Verification items for the finished model (mm, model axes). Face numbers are marked on the shaded views. A direction names the side the tool comes from. Round coordinates to 2 decimals unless told otherwise and drop trailing zeros. Order: outer loops, then holes, each group sorted by start corner. A loop starts at its lowest first (then second) coordinate and runs counter-clockwise, first axis right, second up. Notation, with made-up numbers: (-30.75, -6.75) -> (3.25, -6.75) arc R24 cw to (3.25, 28.25) -> close; hole circle Ø11 at (-26, -2). An arc over 180 degrees is marked (long way). Return JSON: item names as keys, results as strings. Group by question number.
1) Section check C-C on x = 25. Enter the section's corners in (y, z), plus the area to 3 significant figures.
2) Section check D-D on z = 32.5. Enter the section's corners in (x, y), plus the area to 3 significant figures.
3) Scan lines: L1, parallel to X at y = 47, z = 0; L2, parallel to Y at x = -43, z = -38; L3, parallel to X at y = 21, z = 3. Record each from-to range of solid material in increasing order.
4) Section check B-B on y = 12. Enter the section's corners in (x, z).
5) Section check A-A on z = 0. Enter the section's corners in (x, y), plus the area to 3 significant figures.
6) Draft check along Z on the marked faces 1, 2 and 3. Enter one of: pulls with the +Z half, pulls with the -Z half, needs draft (parallel to the pull), parting line crosses it, or undercut.
7) Depth check by flat-ended pin: pin 1 (12 mm diameter, centred on y = 33.5, z = 42.5, fed in from +X); pin 2 (19 mm diameter, centred on x = 68, y = 12.5, fed in from -Z); pin 3 (8 mm diameter, centred on x = 74, z = -18.5, fed in from +Y). Enter the tip coordinate at first touch or a pass-through.
8) Tool access check on the marked faces 4, 5, 6, 7 and 8. Record the directions out of +Z, -Z, +X, -X, +Y, -Y that give a thin tool (end or side, any length) a straight path to the whole face; none if there is none.
```python
from build123d import *

# Parameters (mm, degrees)
SKETCH1_R          = 11
BASE_DEPTH         = 24
SKETCH2_R          = 36
SKETCH2_R_2        = 14
TOP_CYLINDER_DEPTH = 38
SIDE_ARMS_DEPTH    = 56


with BuildPart() as part:
    # Sketch1 → base (new body)
    with BuildSketch(Plane(origin=(0, 0, 0), x_dir=(1, 0, 0), z_dir=(0, 1, 0))):
        with BuildLine():
            Line((-28, -50.793700397), (28, -50.793700397))
            ThreePointArc((28, -50.793700397), (41.012193309, -41.012193309), (50.793700397, -28))
            Line((50.793700397, -28), (88, -28))
            ThreePointArc((88, -28), (116, 0), (88, 28))
            Line((88, 28), (50.793700397, 28))
            ThreePointArc((50.793700397, 28), (41.012193309, 41.012193309), (28, 50.793700397))
            Line((28, 50.793700397), (-28, 50.793700397))
            ThreePointArc((-28, 50.793700397), (-58, 0), (-28, -50.793700397))
        make_face()
        with Locations(Location((88, 0, 0), (0, 0, 270))):
            Circle(SKETCH1_R, mode=Mode.SUBTRACT)
    extrude(amount=BASE_DEPTH)

    # Sketch2 → top cylinder (add)
    with BuildSketch(Plane(origin=(0, 24, 0), x_dir=(1, 0, 0), z_dir=(0, 1, 0))):
        with Locations(Location((0, 0, 0), (0, 0, 270))):
            Circle(SKETCH2_R)
        with Locations(Location((0, 0, 0), (0, 0, 270))):
            Circle(SKETCH2_R_2, mode=Mode.SUBTRACT)
    extrude(amount=TOP_CYLINDER_DEPTH)

    # 3DSketch1 → side arms (add)
    with BuildSketch(Plane(origin=(28, 24, 50.793700397), x_dir=(0, 0, -1), z_dir=(1, 0, 0))):
        Polygon((0, 0), (28.166283399, 23.634318012), (28.166283399, 0), align=None)
        Polygon((101.587400794, 0), (73.421117395, 23.634318012), (73.421117395, 0), align=None)
    extrude(amount=-SIDE_ARMS_DEPTH)


solid = part.part
```
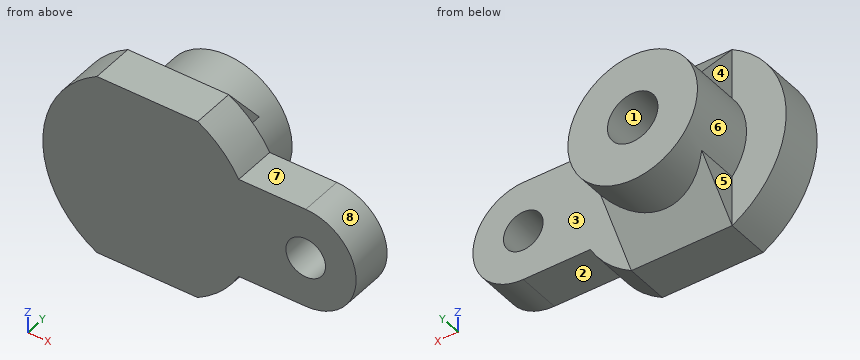
Check result:
{
 "1": {"outline": "(0, -50.79) -> (24, -50.79) -> (44.89, -25.9) -> (62, -25.9) -> (62, 25.9) -> (44.89, 25.9) -> (24, 50.79) -> (0, 50.79) -> close", "area": "4,930 mm^2"},
 "2": {"outline": "(-48.04, 0) -> (48.04, 0) -> (48.04, 24) -> (28, 24) -> (28, 39.35) -> (15.48, 39.35) -> (15.48, 62) -> (-15.48, 62) -> (-15.48, 39.35) -> (-28, 39.35) -> (-28, 24) -> (-48.04, 24) -> close", "area": "3,870 mm^2"},
 "3": {"L1": "-36 to -14, 14 to 36", "L2": "0 to 24", "L3": "-57.92 to 77.42, 98.58 to 115.84"},
 "4": {"outline": "(-28, -50.79) -> (28, -50.79) arc R58 ccw to (50.79, -28) -> (88, -28) arc R28 ccw to (88, 28) -> (50.79, 28) arc R58 ccw to (28, 50.79) -> (-28, 50.79) arc R58 ccw to start; hole circle Ø22 at (88, 0)"},
 "5": {"outline": "(-58, 0) -> (77, 0) -> (77, 24) -> (36, 24) -> (36, 62) -> (14, 62) -> (14, 24) -> (-14, 24) -> (-14, 62) -> (-36, 62) -> (-36, 24) -> (-58, 24) -> close; (99, 0) -> (116, 0) -> (116, 24) -> (99, 24) -> close", "area": "5,320 mm^2"},
 "6": {"face 1": "undercut", "face 2": "pulls with the -Z half", "face 3": "needs draft"},
 "7": {"pin 1": "x = 28", "pin 2": "z = -28", "pin 3": "y = 24"},
 "8": {"face 4": "+Z, -X, +Y", "face 5": "-Z, -X, +Y", "face 6": "+Y", "face 7": "+Z, +X, +Y, -Y", "face 8": "+X, +Y, -Y"}
}
